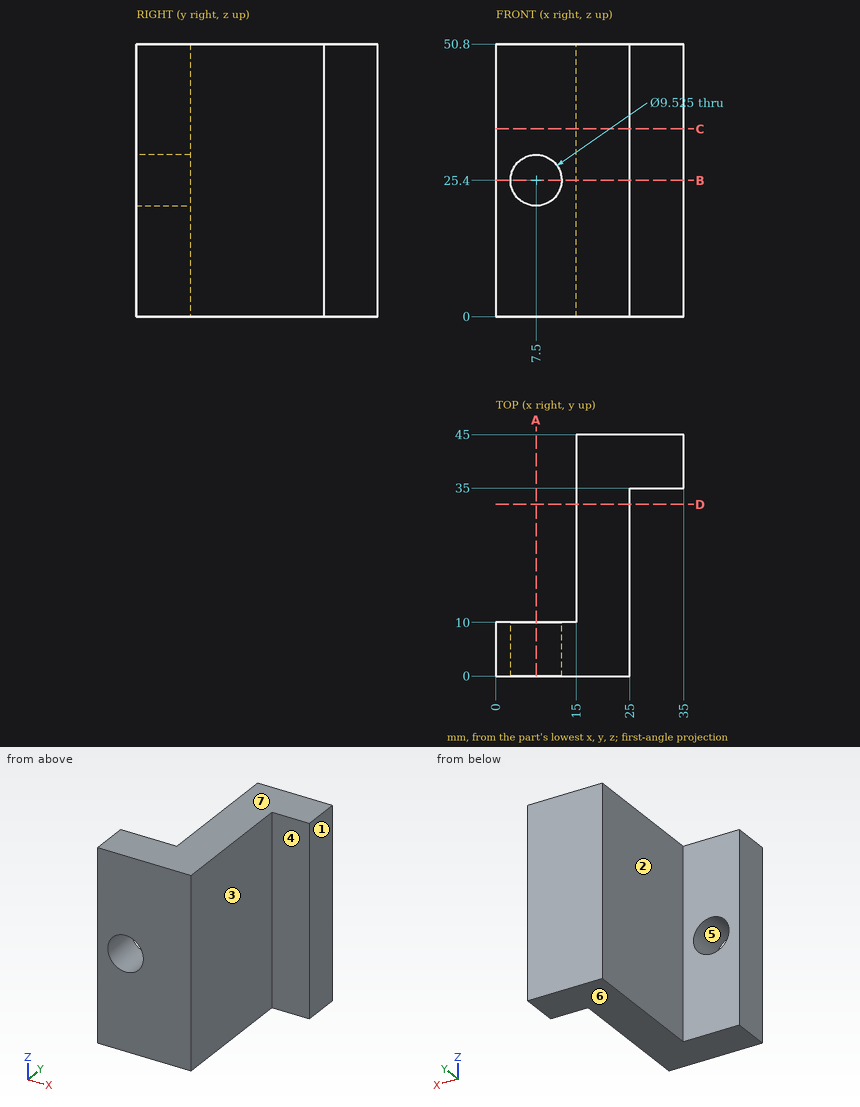
Here's the drawing with two shaded views (mm, measured from the low corner). I have some questions. A direction names the side the tool comes from. Give positions to 0.01 mm unless a question says otherwise; leave off trailing zeros. Order: outer loops, then holes, each group sorted by start corner. A loop starts at its lowest first (then second) coordinate and runs counter-clockwise, first axis right, second up. Notation, with made-up numbers: M 69,55.25 L 85,55.25 A23 ccw 85,83.25 Z; hole C 77,-39.75 d8. An arc over 180 degrees is marked long. One line per question, with ' | ' between items.
Item 1: I'm going to push flat-ended pins straight in: pin 1 Ø5 at (x, z) = (30, 15) entering from -Y; pin 2 Ø10.5 at (y, z) = (25.5, 28) entering from +X; pin 3 Ø4.5 at (x, z) = (8, 35) entering from +Y. Where does each tip first touch, or does it pass through?
Answer block:
pin 1: stops at y = 35 | pin 2: stops at x = 25 | pin 3: stops at y = 10
Item 2: Please list where these lines run through material, in increasing order: L1, parallel to X at y = 7.75, z = 25.4; L2, parallel to Y at x = 28, z = 47; L3, parallel to X at y = 37, z = 26.
Answer block:
L1: x = 0 to 2.74, 12.26 to 25 | L2: y = 35 to 45 | L3: x = 15 to 35
Item 3: Suppose I cut it at A-A, the plane x = 7.5. Write out the boundary of the cut face in (y, z).
Answer block:
outline: M 0,0 L 10,0 L 10,20.64 L 0,20.64 Z; M 0,30.16 L 10,30.16 L 10,50.8 L 0,50.8 Z
Item 4: We'd pull the mould along Z, two halves only. Please class the marked faces 4, 5, 6 and 7: released by +Z, released by -Z, zero draft, split by the parting line, or undercut.
Answer block:
face 4: zero draft | face 5: undercut | face 6: released by -Z | face 7: released by +Z
Item 5: Suppose I cut it at B-B, the plane z = 25.4. Write out the boundary of the cut face in (x, y), then the cut area to 3 significant figures.
Answer block:
outline: M 0,0 L 2.74,0 L 2.74,10 L 0,10 Z; M 12.26,0 L 25,0 L 25,35 L 35,35 L 35,45 L 15,45 L 15,10 L 12.26,10 Z | area: 605 mm2
Item 6: Suppose I cut it at C-C, the plane z = 35. Write out the boundary of the cut face in (x, y), then the cut area to 3 significant figures.
Answer block:
outline: M 0,0 L 25,0 L 25,35 L 35,35 L 35,45 L 15,45 L 15,10 L 0,10 Z | area: 700 mm2
Item 7: For the marked faces 1, 2 and 3, which set-ups out of +Z, -Z, +X, -X, +Y, -Y let a thin tool reach every point of the face, with its end or its side?
Answer block:
face 1: +Z, -Z, +X, +Y, -Y | face 2: +Z, -Z, -X, +Y | face 3: +Z, -Z, +X, -Y
Item 8: Suppose I cut it at D-D, the plane y = 32. Write out the boundary of the cut face in (x, z), then the cut area to 3 significant figures.
Answer block:
outline: M 15,0 L 25,0 L 25,50.8 L 15,50.8 Z | area: 508 mm2
